from build123d import *

# Parameters (mm, degrees)
SKETCH1_W           = 50
SKETCH1_H           = 10
BOSS_EXTRUDE2_DEPTH = 16.65
CUT_EXTRUDE1_START  = -27.3
SKETCH2_R           = 18.45
CUT_EXTRUDE1_DEPTH  = 27.3
SKETCH3_R           = 4
BOSS_EXTRUDE3_DEPTH = 3
CUT_EXTRUDE2_DEPTH  = 3
BOSS_EXTRUDE4_START = 3
SKETCH5_R           = 4
BOSS_EXTRUDE4_DEPTH = 3
SKETCH6_R           = 1.95
BOSS_EXTRUDE5_DEPTH = 3
BOSS_EXTRUDE6_DEPTH = 3
SKETCH9_R           = 3.38
SKETCH9_R_2         = 2.98
CUT_EXTRUDE3_DEPTH  = 1
SKETCH10_R          = 15
CUT_EXTRUDE4_DEPTH  = 61.900656811
FILLET1_R           = 15


with BuildPart() as part:
    # Sketch1 → Boss-Extrude2 (new, symmetric)
    with BuildSketch(Plane(origin=(0, 0, 0), x_dir=(1, 0, 0), z_dir=(0, 1, 0))):
        with Locations((25, 5)):
            Rectangle(SKETCH1_W, SKETCH1_H)
    extrude(amount=BOSS_EXTRUDE2_DEPTH, both=True)

    # Sketch2 → Cut-Extrude1 (cut)
    with BuildSketch(Plane(origin=(0, 13.65, 0), x_dir=(1, 0, 0), z_dir=(0, 1, 0)).offset(CUT_EXTRUDE1_START)):
        Circle(SKETCH2_R)
    extrude(amount=CUT_EXTRUDE1_DEPTH, mode=Mode.SUBTRACT)

    # Sketch3 → Boss-Extrude3 (add)
    with BuildSketch(Plane(origin=(0, 13.65, 0), x_dir=(1, 0, 0), z_dir=(0, 1, 0))):
        Circle(SKETCH3_R)
    extrude(amount=BOSS_EXTRUDE3_DEPTH)

    # Sketch4 → Cut-Extrude2 (cut)
    with BuildSketch(Plane.XZ.offset(-13.65)):
        Polygon((0.869391807, 1.706277494), (0.299572001, 1.891423172), (-0.299572001, 1.891423172), (-0.869391807, 1.706277494), (-1.354109486, 1.354109486), (-1.706277494, 0.869391807), (-1.891423172, 0.299572001), (-1.891423172, -0.299572001), (-1.706277494, -0.869391807), (-1.354109486, -1.354109486), (-0.869391807, -1.706277494), (-0.299572001, -1.891423172), (0.299572001, -1.891423172), (0.869391807, -1.706277494), (1.354109486, -1.354109486), (1.706277494, -0.869391807), (1.891423172, -0.299572001), (1.891423172, 0.299572001), (1.706277494, 0.869391807), (1.354109486, 1.354109486), align=None)
    extrude(amount=-CUT_EXTRUDE2_DEPTH, mode=Mode.SUBTRACT)

    # Sketch5 → Boss-Extrude4 (add)
    with BuildSketch(Plane(origin=(0, -13.65, 0), x_dir=(-1, 0, 0), z_dir=(0, -1, 0)).offset(BOSS_EXTRUDE4_START)):
        Circle(SKETCH5_R)
    extrude(amount=-BOSS_EXTRUDE4_DEPTH)

    # Sketch6 → Boss-Extrude5 (add)
    with BuildSketch(Plane(origin=(0, -13.65, 0), x_dir=(1, 0, 0), z_dir=(0, 1, 0))):
        with Locations(Location((0, 0, 0), (0, 0, 90))):
            Circle(SKETCH6_R)
    extrude(amount=BOSS_EXTRUDE5_DEPTH)

    # Sketch7 → Boss-Extrude6 (add)
    with BuildSketch(Plane(origin=(0, 16.65, 0), x_dir=(1, 0, 0), z_dir=(0, 1, 0))):
        with BuildLine():
            ThreePointArc((2.037195172, -4.526756305), (2.035703314, -4.242437448), (2.220911486, -4.026712227))
            ThreePointArc((2.220911486, -4.026712227), (2.299285714, -3.982479678), (2.376779339, -3.93672188))
            ThreePointArc((2.376779339, -3.93672188), (2.656206947, -3.884189508), (2.901688371, -4.027640924))
            ThreePointArc((2.901688371, -4.027640924), (3.755891391, -4.760966743), (4.811166064, -5.153171946))
            ThreePointArc((4.811166064, -5.153171946), (4.985102807, -4.985102807), (5.153171946, -4.811166064))
            ThreePointArc((5.153171946, -4.811166064), (4.760966743, -3.755891391), (4.027640924, -2.901688371))
            ThreePointArc((4.027640924, -2.901688371), (3.884189508, -2.656206947), (3.93672188, -2.376779339))
            ThreePointArc((3.93672188, -2.376779339), (3.982479678, -2.299285714), (4.026712227, -2.220911486))
            ThreePointArc((4.026712227, -2.220911486), (4.242437448, -2.035703314), (4.526756305, -2.037195172))
            ThreePointArc((4.526756305, -2.037195172), (5.63318073, -2.24517245), (6.743178006, -2.057194784))
            ThreePointArc((6.743178006, -2.057194784), (6.809777075, -1.824674268), (6.868360847, -1.59000606))
            ThreePointArc((6.868360847, -1.59000606), (6.001063841, -0.872213987), (4.938883542, -0.499115381))
            ThreePointArc((4.938883542, -0.499115381), (4.69191026, -0.35824794), (4.597690825, -0.089990347))
            ThreePointArc((4.597690825, -0.089990347), (4.598571429, 0), (4.597690825, 0.089990347))
            ThreePointArc((4.597690825, 0.089990347), (4.69191026, 0.35824794), (4.938883542, 0.499115381))
            ThreePointArc((4.938883542, 0.499115381), (6.001063841, 0.872213987), (6.868360847, 1.59000606))
            ThreePointArc((6.868360847, 1.59000606), (6.809777075, 1.824674268), (6.743178006, 2.057194784))
            ThreePointArc((6.743178006, 2.057194784), (5.63318073, 2.24517245), (4.526756305, 2.037195172))
            ThreePointArc((4.526756305, 2.037195172), (4.242437448, 2.035703314), (4.026712227, 2.220911486))
            ThreePointArc((4.026712227, 2.220911486), (3.982479678, 2.299285714), (3.93672188, 2.376779339))
            ThreePointArc((3.93672188, 2.376779339), (3.884189508, 2.656206947), (4.027640924, 2.901688371))
            ThreePointArc((4.027640924, 2.901688371), (4.760966743, 3.755891391), (5.153171946, 4.811166064))
            ThreePointArc((5.153171946, 4.811166064), (4.985102807, 4.985102807), (4.811166064, 5.153171946))
            ThreePointArc((4.811166064, 5.153171946), (3.755891391, 4.760966743), (2.901688371, 4.027640924))
            ThreePointArc((2.901688371, 4.027640924), (2.656206947, 3.884189508), (2.376779339, 3.93672188))
            ThreePointArc((2.376779339, 3.93672188), (2.299285714, 3.982479678), (2.220911486, 4.026712227))
            ThreePointArc((2.220911486, 4.026712227), (2.035703314, 4.242437448), (2.037195172, 4.526756305))
            ThreePointArc((2.037195172, 4.526756305), (2.24517245, 5.63318073), (2.057194784, 6.743178006))
            ThreePointArc((2.057194784, 6.743178006), (1.824674268, 6.809777075), (1.59000606, 6.868360847))
            ThreePointArc((1.59000606, 6.868360847), (0.872213987, 6.001063841), (0.499115381, 4.938883542))
            ThreePointArc((0.499115381, 4.938883542), (0.35824794, 4.69191026), (0.089990347, 4.597690825))
            ThreePointArc((0.089990347, 4.597690825), (0, 4.598571429), (-0.089990347, 4.597690825))
            ThreePointArc((-0.089990347, 4.597690825), (-0.35824794, 4.69191026), (-0.499115381, 4.938883542))
            ThreePointArc((-0.499115381, 4.938883542), (-0.872213987, 6.001063841), (-1.59000606, 6.868360847))
            ThreePointArc((-1.59000606, 6.868360847), (-1.824674268, 6.809777075), (-2.057194784, 6.743178006))
            ThreePointArc((-2.057194784, 6.743178006), (-2.24517245, 5.63318073), (-2.037195172, 4.526756305))
            ThreePointArc((-2.037195172, 4.526756305), (-2.035703314, 4.242437448), (-2.220911486, 4.026712227))
            ThreePointArc((-2.220911486, 4.026712227), (-2.299285714, 3.982479678), (-2.376779339, 3.93672188))
            ThreePointArc((-2.376779339, 3.93672188), (-2.656206947, 3.884189508), (-2.901688371, 4.027640924))
            ThreePointArc((-2.901688371, 4.027640924), (-3.755891391, 4.760966743), (-4.811166064, 5.153171946))
            ThreePointArc((-4.811166064, 5.153171946), (-4.985102807, 4.985102807), (-5.153171946, 4.811166064))
            ThreePointArc((-5.153171946, 4.811166064), (-4.760966743, 3.755891391), (-4.027640924, 2.901688371))
            ThreePointArc((-4.027640924, 2.901688371), (-3.884189508, 2.656206947), (-3.93672188, 2.376779339))
            ThreePointArc((-3.93672188, 2.376779339), (-3.982479678, 2.299285714), (-4.026712227, 2.220911486))
            ThreePointArc((-4.026712227, 2.220911486), (-4.242437448, 2.035703314), (-4.526756305, 2.037195172))
            ThreePointArc((-4.526756305, 2.037195172), (-5.63318073, 2.24517245), (-6.743178006, 2.057194784))
            ThreePointArc((-6.743178006, 2.057194784), (-6.809777075, 1.824674268), (-6.868360847, 1.59000606))
            ThreePointArc((-6.868360847, 1.59000606), (-6.001063841, 0.872213987), (-4.938883542, 0.499115381))
            ThreePointArc((-4.938883542, 0.499115381), (-4.69191026, 0.35824794), (-4.597690825, 0.089990347))
            ThreePointArc((-4.597690825, 0.089990347), (-4.598571429, 0), (-4.597690825, -0.089990347))
            ThreePointArc((-4.597690825, -0.089990347), (-4.69191026, -0.35824794), (-4.938883542, -0.499115381))
            ThreePointArc((-4.938883542, -0.499115381), (-6.001063841, -0.872213987), (-6.868360847, -1.59000606))
            ThreePointArc((-6.868360847, -1.59000606), (-6.809777075, -1.824674268), (-6.743178006, -2.057194784))
            ThreePointArc((-6.743178006, -2.057194784), (-5.63318073, -2.24517245), (-4.526756305, -2.037195172))
            ThreePointArc((-4.526756305, -2.037195172), (-4.242437448, -2.035703314), (-4.026712227, -2.220911486))
            ThreePointArc((-4.026712227, -2.220911486), (-3.982479678, -2.299285714), (-3.93672188, -2.376779339))
            ThreePointArc((-3.93672188, -2.376779339), (-3.884189508, -2.656206947), (-4.027640924, -2.901688371))
            ThreePointArc((-4.027640924, -2.901688371), (-4.760966743, -3.755891391), (-5.153171946, -4.811166064))
            ThreePointArc((-5.153171946, -4.811166064), (-4.985102807, -4.985102807), (-4.811166064, -5.153171946))
            ThreePointArc((-4.811166064, -5.153171946), (-3.755891391, -4.760966743), (-2.901688371, -4.027640924))
            ThreePointArc((-2.901688371, -4.027640924), (-2.656206947, -3.884189508), (-2.376779339, -3.93672188))
            ThreePointArc((-2.376779339, -3.93672188), (-2.299285714, -3.982479678), (-2.220911486, -4.026712227))
            ThreePointArc((-2.220911486, -4.026712227), (-2.035703314, -4.242437448), (-2.037195172, -4.526756305))
            ThreePointArc((-2.037195172, -4.526756305), (-2.24517245, -5.63318073), (-2.057194784, -6.743178006))
            ThreePointArc((-2.057194784, -6.743178006), (-1.824674268, -6.809777075), (-1.59000606, -6.868360847))
            ThreePointArc((-1.59000606, -6.868360847), (-0.872213987, -6.001063841), (-0.499115381, -4.938883542))
            ThreePointArc((-0.499115381, -4.938883542), (-0.35824794, -4.69191026), (-0.089990347, -4.597690825))
            ThreePointArc((-0.089990347, -4.597690825), (0, -4.598571429), (0.089990347, -4.597690825))
            ThreePointArc((0.089990347, -4.597690825), (0.35824794, -4.69191026), (0.499115381, -4.938883542))
            ThreePointArc((0.499115381, -4.938883542), (0.872213987, -6.001063841), (1.59000606, -6.868360847))
            ThreePointArc((1.59000606, -6.868360847), (1.824674268, -6.809777075), (2.057194784, -6.743178006))
            ThreePointArc((2.057194784, -6.743178006), (2.24517245, -5.63318073), (2.037195172, -4.526756305))
        make_face()
        Polygon((1.706277494, -0.869391807), (1.354109486, -1.354109486), (0.869391807, -1.706277494), (0.299572001, -1.891423172), (-0.299572001, -1.891423172), (-0.869391807, -1.706277494), (-1.354109486, -1.354109486), (-1.706277494, -0.869391807), (-1.891423172, -0.299572001), (-1.891423172, 0.299572001), (-1.706277494, 0.869391807), (-1.354109486, 1.354109486), (-0.869391807, 1.706277494), (-0.299572001, 1.891423172), (0.299572001, 1.891423172), (0.869391807, 1.706277494), (1.354109486, 1.354109486), (1.706277494, 0.869391807), (1.891423172, 0.299572001), (1.891423172, -0.299572001), align=None, mode=Mode.SUBTRACT)
    extrude(amount=-BOSS_EXTRUDE6_DEPTH)

    # Sketch9 → Cut-Extrude3 (cut)
    with BuildSketch(Plane.XZ.offset(-13.65)):
        with Locations(Location((0, 0, 0), (0, 0, 270))):
            Circle(SKETCH9_R)
        with Locations(Location((0, 0, 0), (0, 0, 270))):
            Circle(SKETCH9_R_2, mode=Mode.SUBTRACT)
    extrude(amount=-CUT_EXTRUDE3_DEPTH, mode=Mode.SUBTRACT)

    # Sketch10 → Cut-Extrude4 (cut, through all)
    with BuildSketch(Plane(origin=(0, 16.65, 0), x_dir=(1, 0, 0), z_dir=(0, 1, 0))):
        with Locations((34.225, -6.15)):
            Circle(SKETCH10_R)
    extrude(amount=-CUT_EXTRUDE4_DEPTH, mode=Mode.SUBTRACT)

    # Fillet1
    # the kernel refuses this fillet: 15 mm, written as the material it takes off along each edge
    with BuildSketch(Plane(origin=(50, -52.005339059, -10), x_dir=(-1, 0, 0), z_dir=(0, 1, 0))) as fillet1_piece_1:
        with BuildLine():
            CenterArc((14.142135624, 15), FILLET1_R, 199.471220634, 70.528779366)
            Line((0, 10), (-0.282842712, 9.9))
            ThreePointArc((-0.282842712, 9.9), (-0.3, 5), (-0.3, 0))
            Line((-0.3, 0), (0, -0.3))
            Line((0, -0.3), (14.142135624, -0.3))
            Line((14.142135624, -0.3), (14.142135624, 0))
        make_face()
    extrude(amount=104.010678119, mode=Mode.SUBTRACT)


solid = part.part
The listing builds one solid part. Answer for the finished solid, in the listing's coordinates (mm). A direction names the side the tool comes from. Round coordinates to 2 decimals unless told otherwise and drop trailing zeros. Order: outer loops, then holes, each group sorted by start corner. A loop starts at its lowest first (then second) coordinate and runs counter-clockwise, first axis right, second up. Notation, with made-up numbers: (40.25, -6.5) -> (94.25, -6.5) arc R13 ccw to (94.25, -1.5) -> close; hole circle Ø8 at (-22, 63.25). An arc over 180 degrees is marked (long way). Put each result on its own line as item: value.
Q1. Determine the mould class of faces 6 (the cylindrical face through (-3.77, 15.17, 4.77)), 7 (the flat face through (22, 0, -10)), 8 (the cylindrical face through (-2.734, -15.171, 2.92)), 9 (the cylindrical face through (3.74, 15.17, 4.75)) for opening direction X: pulls with the +X half, pulls with the -X half, needs draft (parallel to the pull), parting line crosses it, or undercut.
Results list:
face 6: undercut
face 7: needs draft
face 8: parting line crosses it
face 9: undercut
Q2. Which of the six approach directions +Z, -Z, +X, -X, +Y, -Y give full straight-line access (tool end or side, diameter ignored) to faces 1 (the cylindrical face through (-2.245, 15.171, -5.649)), 2 (the cylindrical face through (-4.77, 15.17, -3.77)), 3 (the cylindrical face through (-3.74, 15.17, -4.75)), 4 (the cylindrical face through (-3.3, 14.14, 0.73)), 5 (the cylindrical face through (0.864, 15.171, 5.987))?
Results list:
face 1: +Y, -Y
face 2: -X, +Y, -Y
face 3: -Z, +Y, -Y
face 4: none
face 5: +Z, +Y, -Y
Q3. Each of these flat-tipped pins is pushed along its axis until it touches: P1, Ø0.5, axis at y = 15.5, z = 0, coming from the -X side; P2, Ø1.5, axis at y = 3, z = -8.5, coming from the -X side; P3, Ø1, axis at x = 49, y = 2, coming from the +Z side. Where does it stop, or does it pass through?
Results list:
P1: x = -4.63
P2: x = 15.96
P3: z = 0
Q4. Section B-B, the plane y = 6 is taken. Write down the section's boundary in (x, z) (3 decimals).
Results list:
outline: (15.505, -10) -> (35.858, -10) arc R15 ccw to (50, 0) -> (47.906, 0) arc R15 cw to (20.544, 0) -> (18.45, 0) arc R18.45 cw to start
Q5. Consider line 1 along Y through (x, z) = (12, -6); line 2 along X through (y, z) = (-2.5, -1.5); line 3 along X through (y, z) = (-10.5, -5.5). Determine where each line is inside the solid, lowest interval first.
Results list:
line 1: -16.65 to -13.65, 13.65 to 16.65
line 2: 18.39 to 21.32, 47.13 to 49.38
line 3: 17.61 to 24.78, 43.67 to 46.57
Q6. Section A-A, the plane x = 13.5 is taken. Write down the section's boundary in (y, z), and give its area (3 significant figures).
Results list:
outline: (-16.65, -10) -> (-13.65, -10) -> (-13.65, 0) -> (-16.65, 0) -> close; (13.65, -10) -> (16.65, -10) -> (16.65, 0) -> (13.65, 0) -> close
area: 60.0 mm^2
